Part model, mm, in its own coordinate system. Give positions to 0.01 mm unless a question says otherwise; leave off trailing zeros. Loops run counter-clockwise (first coordinate to the right, second up) from the corner with the lowest first, then second, coordinate; pieces in that order, holes last. Notation, with made-up numbers: M -31.5,51.5 L 19.5,51.5 A27 cw 19.5,67.5 Z; hole C -23.75,-2.5 d3. An arc over 180 degrees is marked long. Answer in a Markdown table with one row per item.
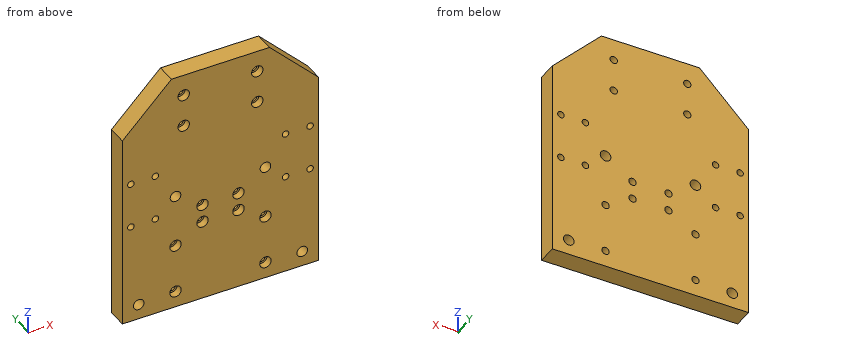
from build123d import *

# Parameters (mm, degrees)
SALIENTE_EXTRUIR1_DEPTH      = 120
SALIENTE_EXTRUIR1_DEPTH_BACK = 120
CROQUIS1_W                   = 300
CROQUIS1_H                   = 24
CORTAR_EXTRUIR1_REACH        = 280.345
CROQUIS2_R                   = 4.5
CROQUIS3_R                   = 7
CORTAR_EXTRUIR2_DEPTH        = 9
CHAFL_N1_SIZE                = 60
CORTAR_EXTRUIR3_REACH        = 280.345
CROQUIS4_R                   = 6.5
CORTAR_EXTRUIR4_REACH        = 280.345
CROQUIS5_R                   = 4
CROQUIS6_R                   = 4.5
CORTAR_EXTRUIR5_DEPTH        = 30
CROQUIS7_R                   = 7
CORTAR_EXTRUIR6_DEPTH        = 9
CORTAR_EXTRUIR7_REACH        = 280.345
CROQUIS8_R                   = 4.5
CROQUIS9_R                   = 7
CORTAR_EXTRUIR8_DEPTH        = 9


with BuildPart() as part:
    # Croquis1 → Saliente-Extruir1 (new, two sides: drawn at the far end of the back side and taken through both)
    with BuildSketch(Plane(origin=(0, 0, 0), x_dir=(0, 0, -1), z_dir=(1, 0, 0)).offset(-SALIENTE_EXTRUIR1_DEPTH_BACK)):
        with Locations((-100, -12)):
            Rectangle(CROQUIS1_W, CROQUIS1_H)
    extrude(amount=SALIENTE_EXTRUIR1_DEPTH + SALIENTE_EXTRUIR1_DEPTH_BACK)

    # Croquis2 → Cortar-Extruir1 (cut, up to next)
    with BuildSketch(Plane(origin=(0, 0, 0), x_dir=(1, 0, 0), z_dir=(0, 1, 0)), mode=Mode.PRIVATE) as cortar_extruir1_sk1:
        with Locations(Location((45, -183.8, 0), (0, 0, 270))):
            Circle(CROQUIS2_R)
    cortar_extruir1_tool1 = extrude(cortar_extruir1_sk1.sketch, amount=-CORTAR_EXTRUIR1_REACH, mode=Mode.PRIVATE) & part.part
    # Croquis2 → Cortar-Extruir1 (cut, up to next)
    with BuildSketch(Plane(origin=(0, 0, 0), x_dir=(1, 0, 0), z_dir=(0, 1, 0)), mode=Mode.PRIVATE) as cortar_extruir1_sk2:
        with Locations(Location((45, -223.8, 0), (0, 0, 270))):
            Circle(CROQUIS2_R)
    cortar_extruir1_tool2 = extrude(cortar_extruir1_sk2.sketch, amount=-CORTAR_EXTRUIR1_REACH, mode=Mode.PRIVATE) & part.part
    # Croquis2 → Cortar-Extruir1 (cut, up to next)
    with BuildSketch(Plane(origin=(0, 0, 0), x_dir=(1, 0, 0), z_dir=(0, 1, 0)), mode=Mode.PRIVATE) as cortar_extruir1_sk3:
        with Locations(Location((-45, -183.8, 0), (0, 0, 270))):
            Circle(CROQUIS2_R)
    cortar_extruir1_tool3 = extrude(cortar_extruir1_sk3.sketch, amount=-CORTAR_EXTRUIR1_REACH, mode=Mode.PRIVATE) & part.part
    # Croquis2 → Cortar-Extruir1 (cut, up to next)
    with BuildSketch(Plane(origin=(0, 0, 0), x_dir=(1, 0, 0), z_dir=(0, 1, 0)), mode=Mode.PRIVATE) as cortar_extruir1_sk4:
        with Locations(Location((-45, -223.8, 0), (0, 0, 270))):
            Circle(CROQUIS2_R)
    cortar_extruir1_tool4 = extrude(cortar_extruir1_sk4.sketch, amount=-CORTAR_EXTRUIR1_REACH, mode=Mode.PRIVATE) & part.part
    add(cortar_extruir1_tool1.solids().sort_by_distance((45, 0, 183.8))[0], mode=Mode.SUBTRACT)
    add(cortar_extruir1_tool2.solids().sort_by_distance((45, 0, 223.8))[0], mode=Mode.SUBTRACT)
    add(cortar_extruir1_tool3.solids().sort_by_distance((-45, 0, 183.8))[0], mode=Mode.SUBTRACT)
    add(cortar_extruir1_tool4.solids().sort_by_distance((-45, 0, 223.8))[0], mode=Mode.SUBTRACT)

    # Croquis3 → Cortar-Extruir2 (cut)
    with BuildSketch(Plane.XZ.offset(24)):
        with Locations(Location((-45, 223.8, 0), (0, 0, 270))):
            Circle(CROQUIS3_R)
        with Locations(Location((-45, 183.8, 0), (0, 0, 270))):
            Circle(CROQUIS3_R)
        with Locations(Location((45, 223.8, 0), (0, 0, 270))):
            Circle(CROQUIS3_R)
        with Locations(Location((45, 183.8, 0), (0, 0, 270))):
            Circle(CROQUIS3_R)
    extrude(amount=-CORTAR_EXTRUIR2_DEPTH, mode=Mode.SUBTRACT)

    # Chafl_n1
    chafl_n1_edges = [part.edges().sort_by_distance(p)[0] for p in [
        (-120, -12, 250),
        (120, -12, 250),
    ]]
    chamfer(chafl_n1_edges, length=CHAFL_N1_SIZE)

    # Croquis4 → Cortar-Extruir3 (cut, up to next)
    with BuildSketch(Plane(origin=(0, 0, 0), x_dir=(1, 0, 0), z_dir=(0, 1, 0)), mode=Mode.PRIVATE) as cortar_extruir3_sk1:
        with Locations(Location((100, 31.5, 0), (0, 0, 270))):
            Circle(CROQUIS4_R)
    cortar_extruir3_tool1 = extrude(cortar_extruir3_sk1.sketch, amount=-CORTAR_EXTRUIR3_REACH, mode=Mode.PRIVATE) & part.part
    # Croquis4 → Cortar-Extruir3 (cut, up to next)
    with BuildSketch(Plane(origin=(0, 0, 0), x_dir=(1, 0, 0), z_dir=(0, 1, 0)), mode=Mode.PRIVATE) as cortar_extruir3_sk2:
        with Locations(Location((-100, 31.5, 0), (0, 0, 270))):
            Circle(CROQUIS4_R)
    cortar_extruir3_tool2 = extrude(cortar_extruir3_sk2.sketch, amount=-CORTAR_EXTRUIR3_REACH, mode=Mode.PRIVATE) & part.part
    # Croquis4 → Cortar-Extruir3 (cut, up to next)
    with BuildSketch(Plane(origin=(0, 0, 0), x_dir=(1, 0, 0), z_dir=(0, 1, 0)), mode=Mode.PRIVATE) as cortar_extruir3_sk3:
        with Locations(Location((55, -94.5, 0), (0, 0, 270))):
            Circle(CROQUIS4_R)
    cortar_extruir3_tool3 = extrude(cortar_extruir3_sk3.sketch, amount=-CORTAR_EXTRUIR3_REACH, mode=Mode.PRIVATE) & part.part
    # Croquis4 → Cortar-Extruir3 (cut, up to next)
    with BuildSketch(Plane(origin=(0, 0, 0), x_dir=(1, 0, 0), z_dir=(0, 1, 0)), mode=Mode.PRIVATE) as cortar_extruir3_sk4:
        with Locations(Location((-55, -94.5, 0), (0, 0, 270))):
            Circle(CROQUIS4_R)
    cortar_extruir3_tool4 = extrude(cortar_extruir3_sk4.sketch, amount=-CORTAR_EXTRUIR3_REACH, mode=Mode.PRIVATE) & part.part
    add(cortar_extruir3_tool1.solids().sort_by_distance((100, 0, -31.5))[0], mode=Mode.SUBTRACT)
    add(cortar_extruir3_tool2.solids().sort_by_distance((-100, 0, -31.5))[0], mode=Mode.SUBTRACT)
    add(cortar_extruir3_tool3.solids().sort_by_distance((55, 0, 94.5))[0], mode=Mode.SUBTRACT)
    add(cortar_extruir3_tool4.solids().sort_by_distance((-55, 0, 94.5))[0], mode=Mode.SUBTRACT)

    # Croquis5 → Cortar-Extruir4 (cut, up to next)
    with BuildSketch(Plane(origin=(0, 0, 0), x_dir=(1, 0, 0), z_dir=(0, 1, 0)), mode=Mode.PRIVATE) as cortar_extruir4_sk1:
        with Locations(Location((79.6, -129.6, 0), (0, 0, 270))):
            Circle(CROQUIS5_R)
    cortar_extruir4_tool1 = extrude(cortar_extruir4_sk1.sketch, amount=-CORTAR_EXTRUIR4_REACH, mode=Mode.PRIVATE) & part.part
    # Croquis5 → Cortar-Extruir4 (cut, up to next)
    with BuildSketch(Plane(origin=(0, 0, 0), x_dir=(1, 0, 0), z_dir=(0, 1, 0)), mode=Mode.PRIVATE) as cortar_extruir4_sk2:
        with Locations(Location((109.6, -129.6, 0), (0, 0, 270))):
            Circle(CROQUIS5_R)
    cortar_extruir4_tool2 = extrude(cortar_extruir4_sk2.sketch, amount=-CORTAR_EXTRUIR4_REACH, mode=Mode.PRIVATE) & part.part
    # Croquis5 → Cortar-Extruir4 (cut, up to next)
    with BuildSketch(Plane(origin=(0, 0, 0), x_dir=(1, 0, 0), z_dir=(0, 1, 0)), mode=Mode.PRIVATE) as cortar_extruir4_sk3:
        with Locations(Location((109.6, -73.6, 0), (0, 0, 270))):
            Circle(CROQUIS5_R)
    cortar_extruir4_tool3 = extrude(cortar_extruir4_sk3.sketch, amount=-CORTAR_EXTRUIR4_REACH, mode=Mode.PRIVATE) & part.part
    # Croquis5 → Cortar-Extruir4 (cut, up to next)
    with BuildSketch(Plane(origin=(0, 0, 0), x_dir=(1, 0, 0), z_dir=(0, 1, 0)), mode=Mode.PRIVATE) as cortar_extruir4_sk4:
        with Locations(Location((79.6, -73.6, 0), (0, 0, 270))):
            Circle(CROQUIS5_R)
    cortar_extruir4_tool4 = extrude(cortar_extruir4_sk4.sketch, amount=-CORTAR_EXTRUIR4_REACH, mode=Mode.PRIVATE) & part.part
    # Croquis5 → Cortar-Extruir4 (cut, up to next)
    with BuildSketch(Plane(origin=(0, 0, 0), x_dir=(1, 0, 0), z_dir=(0, 1, 0)), mode=Mode.PRIVATE) as cortar_extruir4_sk5:
        with Locations(Location((-109.6, -129.6, 0), (0, 0, 270))):
            Circle(CROQUIS5_R)
    cortar_extruir4_tool5 = extrude(cortar_extruir4_sk5.sketch, amount=-CORTAR_EXTRUIR4_REACH, mode=Mode.PRIVATE) & part.part
    # Croquis5 → Cortar-Extruir4 (cut, up to next)
    with BuildSketch(Plane(origin=(0, 0, 0), x_dir=(1, 0, 0), z_dir=(0, 1, 0)), mode=Mode.PRIVATE) as cortar_extruir4_sk6:
        with Locations(Location((-79.6, -129.6, 0), (0, 0, 270))):
            Circle(CROQUIS5_R)
    cortar_extruir4_tool6 = extrude(cortar_extruir4_sk6.sketch, amount=-CORTAR_EXTRUIR4_REACH, mode=Mode.PRIVATE) & part.part
    # Croquis5 → Cortar-Extruir4 (cut, up to next)
    with BuildSketch(Plane(origin=(0, 0, 0), x_dir=(1, 0, 0), z_dir=(0, 1, 0)), mode=Mode.PRIVATE) as cortar_extruir4_sk7:
        with Locations(Location((-109.6, -73.6, 0), (0, 0, 270))):
            Circle(CROQUIS5_R)
    cortar_extruir4_tool7 = extrude(cortar_extruir4_sk7.sketch, amount=-CORTAR_EXTRUIR4_REACH, mode=Mode.PRIVATE) & part.part
    # Croquis5 → Cortar-Extruir4 (cut, up to next)
    with BuildSketch(Plane(origin=(0, 0, 0), x_dir=(1, 0, 0), z_dir=(0, 1, 0)), mode=Mode.PRIVATE) as cortar_extruir4_sk8:
        with Locations(Location((-79.6, -73.6, 0), (0, 0, 270))):
            Circle(CROQUIS5_R)
    cortar_extruir4_tool8 = extrude(cortar_extruir4_sk8.sketch, amount=-CORTAR_EXTRUIR4_REACH, mode=Mode.PRIVATE) & part.part
    add(cortar_extruir4_tool1.solids().sort_by_distance((79.6, 0, 129.6))[0], mode=Mode.SUBTRACT)
    add(cortar_extruir4_tool2.solids().sort_by_distance((109.6, 0, 129.6))[0], mode=Mode.SUBTRACT)
    add(cortar_extruir4_tool3.solids().sort_by_distance((109.6, 0, 73.6))[0], mode=Mode.SUBTRACT)
    add(cortar_extruir4_tool4.solids().sort_by_distance((79.6, 0, 73.6))[0], mode=Mode.SUBTRACT)
    add(cortar_extruir4_tool5.solids().sort_by_distance((-109.6, 0, 129.6))[0], mode=Mode.SUBTRACT)
    add(cortar_extruir4_tool6.solids().sort_by_distance((-79.6, 0, 129.6))[0], mode=Mode.SUBTRACT)
    add(cortar_extruir4_tool7.solids().sort_by_distance((-109.6, 0, 73.6))[0], mode=Mode.SUBTRACT)
    add(cortar_extruir4_tool8.solids().sort_by_distance((-79.6, 0, 73.6))[0], mode=Mode.SUBTRACT)

    # Croquis6 → Cortar-Extruir5 (cut)
    with BuildSketch(Plane(origin=(0, 0, 0), x_dir=(1, 0, 0), z_dir=(0, 1, 0))):
        with Locations(Location((-55, -30, 0), (0, 0, 270))):
            Circle(CROQUIS6_R)
        with Locations(Location((-55, 30, 0), (0, 0, 270))):
            Circle(CROQUIS6_R)
        with Locations(Location((55, 30, 0), (0, 0, 270))):
            Circle(CROQUIS6_R)
        with Locations(Location((55, -30, 0), (0, 0, 270))):
            Circle(CROQUIS6_R)
    extrude(amount=-CORTAR_EXTRUIR5_DEPTH, mode=Mode.SUBTRACT)

    # Croquis7 → Cortar-Extruir6 (cut)
    with BuildSketch(Plane.XZ.offset(24)):
        with Locations(Location((55, 30, 0), (0, 0, 270))):
            Circle(CROQUIS7_R)
        with Locations(Location((55, -30, 0), (0, 0, 270))):
            Circle(CROQUIS7_R)
        with Locations(Location((-55, 30, 0), (0, 0, 270))):
            Circle(CROQUIS7_R)
        with Locations(Location((-55, -30, 0), (0, 0, 270))):
            Circle(CROQUIS7_R)
    extrude(amount=-CORTAR_EXTRUIR6_DEPTH, mode=Mode.SUBTRACT)

    # Croquis8 → Cortar-Extruir7 (cut, up to next)
    with BuildSketch(Plane(origin=(0, 0, 0), x_dir=(1, 0, 0), z_dir=(0, 1, 0)), mode=Mode.PRIVATE) as cortar_extruir7_sk1:
        with Locations(Location((-22, -50, 0), (0, 0, 270))):
            Circle(CROQUIS8_R)
    cortar_extruir7_tool1 = extrude(cortar_extruir7_sk1.sketch, amount=-CORTAR_EXTRUIR7_REACH, mode=Mode.PRIVATE) & part.part
    # Croquis8 → Cortar-Extruir7 (cut, up to next)
    with BuildSketch(Plane(origin=(0, 0, 0), x_dir=(1, 0, 0), z_dir=(0, 1, 0)), mode=Mode.PRIVATE) as cortar_extruir7_sk2:
        with Locations(Location((-22, -72, 0), (0, 0, 270))):
            Circle(CROQUIS8_R)
    cortar_extruir7_tool2 = extrude(cortar_extruir7_sk2.sketch, amount=-CORTAR_EXTRUIR7_REACH, mode=Mode.PRIVATE) & part.part
    # Croquis8 → Cortar-Extruir7 (cut, up to next)
    with BuildSketch(Plane(origin=(0, 0, 0), x_dir=(1, 0, 0), z_dir=(0, 1, 0)), mode=Mode.PRIVATE) as cortar_extruir7_sk3:
        with Locations(Location((22, -72, 0), (0, 0, 270))):
            Circle(CROQUIS8_R)
    cortar_extruir7_tool3 = extrude(cortar_extruir7_sk3.sketch, amount=-CORTAR_EXTRUIR7_REACH, mode=Mode.PRIVATE) & part.part
    # Croquis8 → Cortar-Extruir7 (cut, up to next)
    with BuildSketch(Plane(origin=(0, 0, 0), x_dir=(1, 0, 0), z_dir=(0, 1, 0)), mode=Mode.PRIVATE) as cortar_extruir7_sk4:
        with Locations(Location((22, -50, 0), (0, 0, 270))):
            Circle(CROQUIS8_R)
    cortar_extruir7_tool4 = extrude(cortar_extruir7_sk4.sketch, amount=-CORTAR_EXTRUIR7_REACH, mode=Mode.PRIVATE) & part.part
    add(cortar_extruir7_tool1.solids().sort_by_distance((-22, 0, 50))[0], mode=Mode.SUBTRACT)
    add(cortar_extruir7_tool2.solids().sort_by_distance((-22, 0, 72))[0], mode=Mode.SUBTRACT)
    add(cortar_extruir7_tool3.solids().sort_by_distance((22, 0, 72))[0], mode=Mode.SUBTRACT)
    add(cortar_extruir7_tool4.solids().sort_by_distance((22, 0, 50))[0], mode=Mode.SUBTRACT)

    # Croquis9 → Cortar-Extruir8 (cut)
    with BuildSketch(Plane.XZ.offset(24)):
        with Locations(Location((22, 50, 0), (0, 0, 270))):
            Circle(CROQUIS9_R)
        with Locations(Location((22, 72, 0), (0, 0, 270))):
            Circle(CROQUIS9_R)
        with Locations(Location((-22, 72, 0), (0, 0, 270))):
            Circle(CROQUIS9_R)
        with Locations(Location((-22, 50, 0), (0, 0, 270))):
            Circle(CROQUIS9_R)
    extrude(amount=-CORTAR_EXTRUIR8_DEPTH, mode=Mode.SUBTRACT)


solid = part.part
(1) Saw through at C-C (y = -20). Give the number of separate pieces and of enclosed holes in the cut face, plus the area to 3 significant figures.
Recorded:
| item | result |
|---|---|
| separate pieces | 1 |
| enclosed holes | 24 |
| area | 65,600 mm^2 |
(2) Saw through at B-B (z = 129.6). Write the cut outline in (x, y), plus the area to 3 significant figures.
Recorded:
| item | result |
|---|---|
| outline | M -120,-24 L -113.6,-24 L -113.6,0 L -120,0 Z; M -105.6,-24 L -83.6,-24 L -83.6,0 L -105.6,0 Z; M -75.6,-24 L 75.6,-24 L 75.6,0 L -75.6,0 Z; M 83.6,-24 L 105.6,-24 L 105.6,0 L 83.6,0 Z; M 113.6,-24 L 120,-24 L 120,0 L 113.6,0 Z |
| area | 4,990 mm^2 |
(3) Saw through at A-A (x = 109.6). Write the cut outline in (y, z), plus the area to 3 significant figures.
Recorded:
| item | result |
|---|---|
| outline | M -24,-50 L 0,-50 L 0,69.6 L -24,69.6 Z; M -24,77.6 L 0,77.6 L 0,125.6 L -24,125.6 Z; M -24,133.6 L 0,133.6 L 0,200.4 L -24,200.4 Z |
| area | 5,630 mm^2 |
(4) Drill centre lines: line 1 along Z through (x, y) = (-21.5, -2.25); line 2 along X through (y, z) = (-13.5, 129.6); line 3 along X through (y, z) = (-17.25, 94.5). Where is each one in solid material? Low to high.
Recorded:
| item | result |
|---|---|
| line 1 | z = -50 to 45.53, 54.47 to 67.53, 76.47 to 250 |
| line 2 | x = -120 to -113.6, -105.6 to -83.6, -75.6 to 75.6, 83.6 to 105.6, 113.6 to 120 |
| line 3 | x = -120 to -61.5, -48.5 to 48.5, 61.5 to 120 |
(5) Pin check, flat tips, straight feed: pin 1 Ø5 at (x, z) = (79.6, 129.6) entering from -Y; pin 2 Ø22.5 at (x, z) = (22, 72) entering from +Y; pin 3 Ø6 at (x, y) = (64, -6.5) entering from +Z; pin 4 Ø4 at (x, z) = (-42, 224) entering from -Y. Stop position of each tip, or through.
Recorded:
| item | result |
|---|---|
| pin 1 | passes through |
| pin 2 | stops at y = 0 |
| pin 3 | stops at z = 249 |
| pin 4 | stops at y = -15 |
(6) Saw through at D-D (z = 30). Write the cut outline in (x, y).
Recorded:
| item | result |
|---|---|
| outline | M -120,-24 L -62,-24 L -62,-15 L -59.5,-15 L -59.5,0 L -120,0 Z; M -50.5,-15 L -48,-15 L -48,-24 L 48,-24 L 48,-15 L 50.5,-15 L 50.5,0 L -50.5,0 Z; M 59.5,-15 L 62,-15 L 62,-24 L 120,-24 L 120,0 L 59.5,0 Z |
